Verification items for this drawing (mm, ordinates from the low corner). Give positions to 0.01 mm unless a question says otherwise; leave off trailing zeros. Loops run counter-clockwise (first coordinate to the right, second up) from the corner with the lowest first, then second, coordinate; pieces in that order, holes last. Notation, with made-up numbers: M -11,-4 L 2,-4 A22 ccw 2,35 Z; hole C 30.25,-19 d5. An arc over 180 degrees is marked long. Answer in a Markdown table with one row per item.
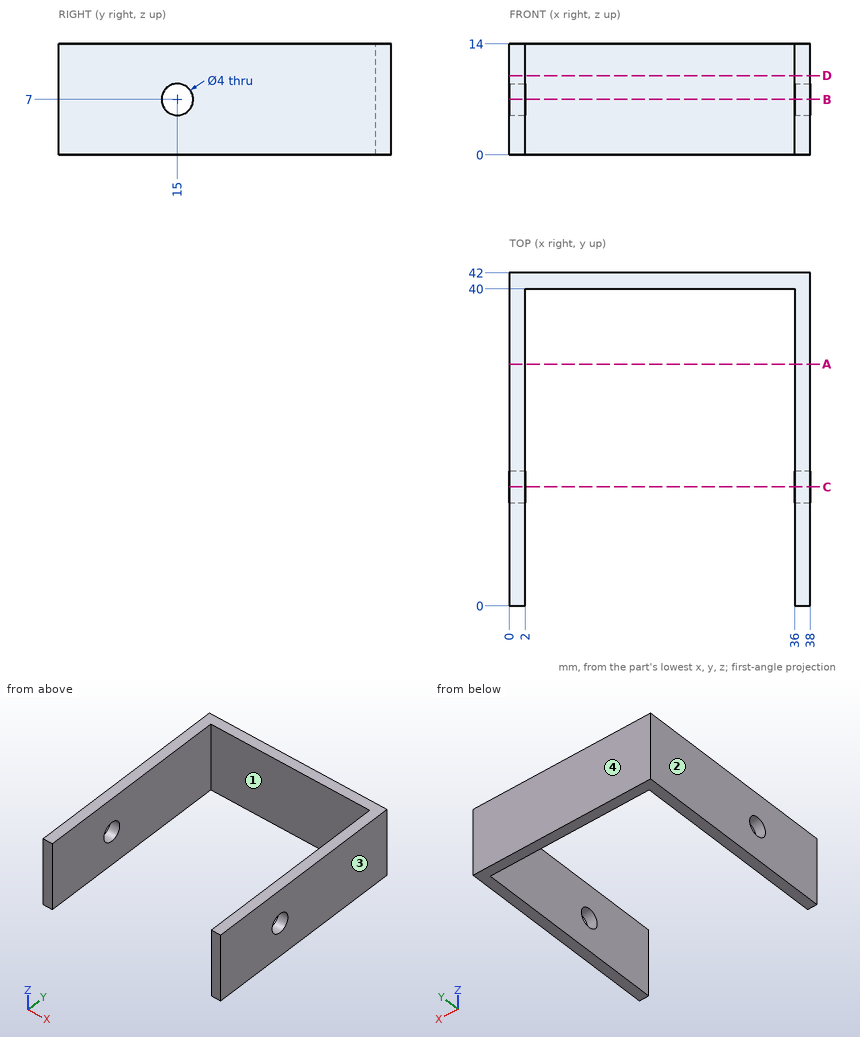
Item 1: Go/stop test with a flat-tipped pin: pin 1 (4 mm diameter, centred on x = 12.5, z = 11.5, fed in from -Y). Record where the tip stops, or that it passes through.
Reported:
| item | result |
|---|---|
| pin 1 | stops at y = 40 |
Item 2: Release check for a two-part mould opening along X. For the marked faces 1, 2, 3 and 4 record: released by +X, released by -X, zero draft, split by the parting line, or undercut.
Reported:
| item | result |
|---|---|
| face 1 | undercut |
| face 2 | released by -X |
| face 3 | released by +X |
| face 4 | zero draft |
Item 3: Scan lines: L1, parallel to X at y = 6, z = 5.5; L2, parallel to Z at x = 36.4, y = 15; L3, parallel to Y at x = 34, z = 8. Record each from-to range of solid material in increasing order. Write a range as [from, to].
Reported:
| item | result |
|---|---|
| L1 | x = [0, 2], [36, 38] |
| L2 | z = [0, 5], [9, 14] |
| L3 | y = [40, 42] |
Item 4: Sectioned sample at C-C (y = 15). Record the cut outline in (x, z).
Reported:
| item | result |
|---|---|
| outline | M 0,0 L 2,0 L 2,5 L 0,5 Z; M 0,9 L 2,9 L 2,14 L 0,14 Z; M 36,0 L 38,0 L 38,5 L 36,5 Z; M 36,9 L 38,9 L 38,14 L 36,14 Z |
Item 5: Sectioned sample at D-D (z = 10). Record the cut outline in (x, y), and give its area (3 significant figures).
Reported:
| item | result |
|---|---|
| outline | M 0,0 L 2,0 L 2,40 L 36,40 L 36,0 L 38,0 L 38,42 L 0,42 Z |
| area | 236 mm^2 |
Item 6: Sectioned sample at B-B (z = 7). Record the cut outline in (x, y), and give its area (3 significant figures).
Reported:
| item | result |
|---|---|
| outline | M 0,0 L 2,0 L 2,13 L 0,13 Z; M 0,17 L 2,17 L 2,40 L 36,40 L 36,17 L 38,17 L 38,42 L 0,42 Z; M 36,0 L 38,0 L 38,13 L 36,13 Z |
| area | 220 mm^2 |
Item 7: Sectioned sample at A-A (y = 30.5). Record the cut outline in (x, z).
Reported:
| item | result |
|---|---|
| outline | M 0,0 L 2,0 L 2,14 L 0,14 Z; M 36,0 L 38,0 L 38,14 L 36,14 Z |
